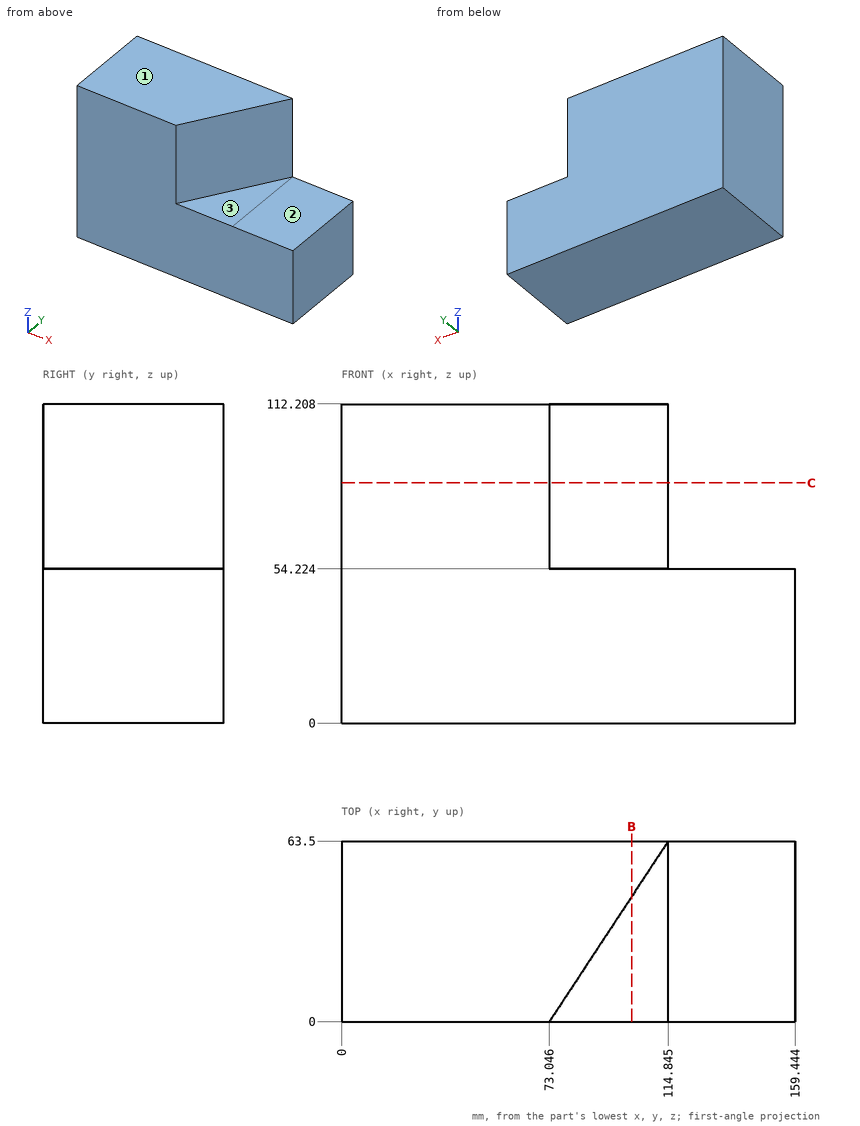
Geometry check sheet. Reference: drawing and pictorial views, mm from the part's lowest x, y, z. A direction names the side the tool comes from. Give positions to 0.01 mm unless a question says otherwise; leave off trailing zeros. Order: outer loops, then holes, each group sorted by start corner. A loop starts at its lowest first (then second) coordinate and runs counter-clockwise, first axis right, second up. Notation, with made-up numbers: M -21.75,55.25 L 19.25,55.25 A31 cw 19.25,88.25 Z; hole C 59,81.25 d10. An arc over 180 degrees is marked long. Answer in a Markdown table with one row per item. Add a question column.
Q1. Access from +Z, -Z, +X, -X, +Y, -Y to the whole of each face (thin tool, end or side, straight path). Record for the marked faces 1, 2 and 3.
Q2. Gauge pin test, flat ends, axial feed: pin 1 Ø2 at (y, z) = (39, 23) entering from -X; pin 2 Ø1 at (y, z) = (28, 85) entering from +X (1 decimal); pin 3 Ø8 at (y, z) = (19, 98) entering from +X (1 decimal). Record the tip position at first contact, or that the pin passes through.
Q3. Thickness scan on L1, parallel to Z at x = 146, y = 19; L2, parallel to X at y = 59.5, z = 99.5; L3, parallel to X at y = 54, z = 94.5. Record the ranges inside material, lowest first.
Q4. Sectioned sample at C-C, the plane z = 84.5. Record the boundary of the cut face in (x, y) (1 decimal).
Q5. Sectioned sample at B-B, the plane x = 102. Record the boundary of the cut face in (y, z).
Verdict:
| question | item | result |
|---|---|---|
| 1 | face 1 | +Z, +X, -X, +Y, -Y |
| 1 | face 2 | +Z, +X, +Y, -Y |
| 1 | face 3 | +Z, +X, -Y |
| 2 | pin 1 | x = 0 |
| 2 | pin 2 | x = 91.8 |
| 2 | pin 3 | x = 88.2 |
| 3 | L1 | 0 to 54.22 |
| 3 | L2 | 0 to 112.21 |
| 3 | L3 | 0 to 108.59 |
| 4 | outline | M 0,0 L 73,0 L 114.8,63.5 L 0,63.5 Z |
| 5 | outline | M 0,0 L 63.5,0 L 63.5,112.21 L 43.99,112.21 L 43.99,54.22 L 0,54.22 Z |
